from build123d import *

# Parameters (mm, degrees)
F1_DEPTH = 5
F2_R     = 1.3
F3_DEPTH = 110
F4_R     = 1


with BuildPart() as f1:
    # F0 (on Front) → F1 (new body, symmetric)
    with BuildSketch(Plane.XZ):
        Polygon((-55, 12), (-55, 0), (0, 0), (55, 0), (55, 12), (52.5, 12), (47, 3.5), (0, 3.5), (-47, 3.5), (-52.5, 12), align=None)
    extrude(amount=F1_DEPTH, both=True)

    # F2 (on face) → F3 (cut, through all)
    with BuildSketch(Plane(origin=(-55, 0, 0), x_dir=(0, -1, 0), z_dir=(-1, 0, 0))):
        with Locations((0, 6.7)):
            Circle(F2_R)
    extrude(amount=-F3_DEPTH, mode=Mode.SUBTRACT)

    # F4
    f4_edges = [f1.edges().sort_by_distance(p)[0] for p in [
        (-49.75, 5, 7.75),
        (-49.75, -5, 7.75),
        (0, -5, 3.5),
        (0, 5, 3.5),
        (49.75, 5, 7.75),
        (49.75, -5, 7.75),
        (-55, -5, 6),
        (-55, 5, 6),
        (55, -5, 6),
        (55, 5, 6),
    ]]
    fillet(f4_edges, radius=F4_R)


solid = f1.part
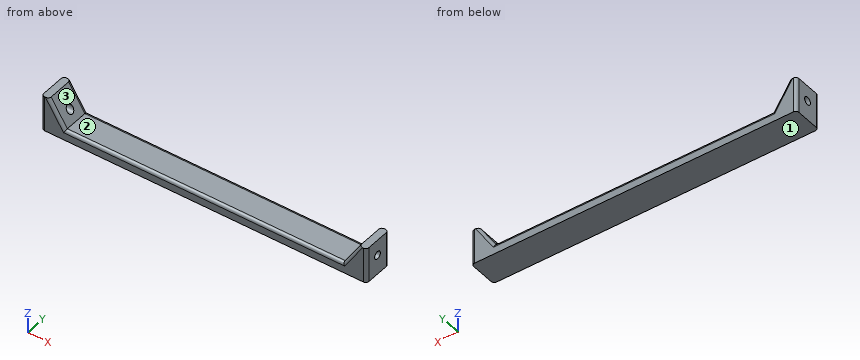
Work out the finished part from the listing and answer in its coordinate system (mm). Face numbers are marked on the shaded views. Coordinates: 2 decimals unless noted, no trailing zeros. Write each loop counter-clockwise with the first axis right and the second up, starting at its lowest first coordinate (ties: lowest second). Pieces come first, ordered by that corner, then holes. Notation, with made-up numbers: M 46,51.5 L 100,51.5 A20 ccw 100,70.5 Z; hole C 9.25,59 d5. An arc over 180 degrees is marked long. Answer as CSV lines item,"result". Start each with the question number.
Item 1: Section B-B on x = -38.5 is taken. Write down the section's boundary in (y, z), and give its area (3 significant figures).
Item 2: Section C-C on z = 6.7 is taken. Give the number of separate pieces and of enclosed holes in the cut face, and give its area (3 significant figures).
Item 3: Consider L1, parallel to Z at x = 53.5, y = 0; L2, parallel to Y at x = 53, z = 6.7; L3, parallel to X at y = -0.75, z = 10. Determine where each line is inside the solid, lowest interval first.
Item 4: Determine the mould class of the marked faces 1, 2 and 3 for opening direction X: released by +X, released by -X, zero draft, split by the parting line, or undercut.
Item 5: A flat-ended cylindrical pin translates along its axis: P1, Ø4, axis at x = -4.5, y = 1, coming from the +Z side. Find the tip coordinate at first contact, or state that the pin passes through.
Item 6: Section A-A on y = 0 is taken. Write down the section's boundary in (x, z), and give its area (3 significant figures).
Checks:
1,outline,"M -5,0 L 5,0 L 5,2.5 A1 ccw 4,3.5 L -4,3.5 A1 ccw -5,2.5 Z"
1,area,"34.6 mm²"
2,separate pieces,"4"
2,enclosed holes,"0"
2,area,"85.9 mm²"
3,L1,"z = 0 to 5.4, 8 to 12"
3,L2,"y = -5 to -1.3, 1.3 to 5"
3,L3,"x = -55 to -51.21, 51.21 to 55"
4,face 1,"zero draft"
4,face 2,"undercut"
4,face 3,"undercut"
5,P1,"stops at z = 3.5"
6,outline,"M -55,0 L 55,0 L 55,5.4 L 48.23,5.4 L 47,3.5 L -47,3.5 L -48.23,5.4 L -55,5.4 Z; M -55,8 L -49.91,8 L -52.5,12 L -55,12 Z; M 49.91,8 L 55,8 L 55,12 L 52.5,12 Z"
6,area,"443 mm²"
